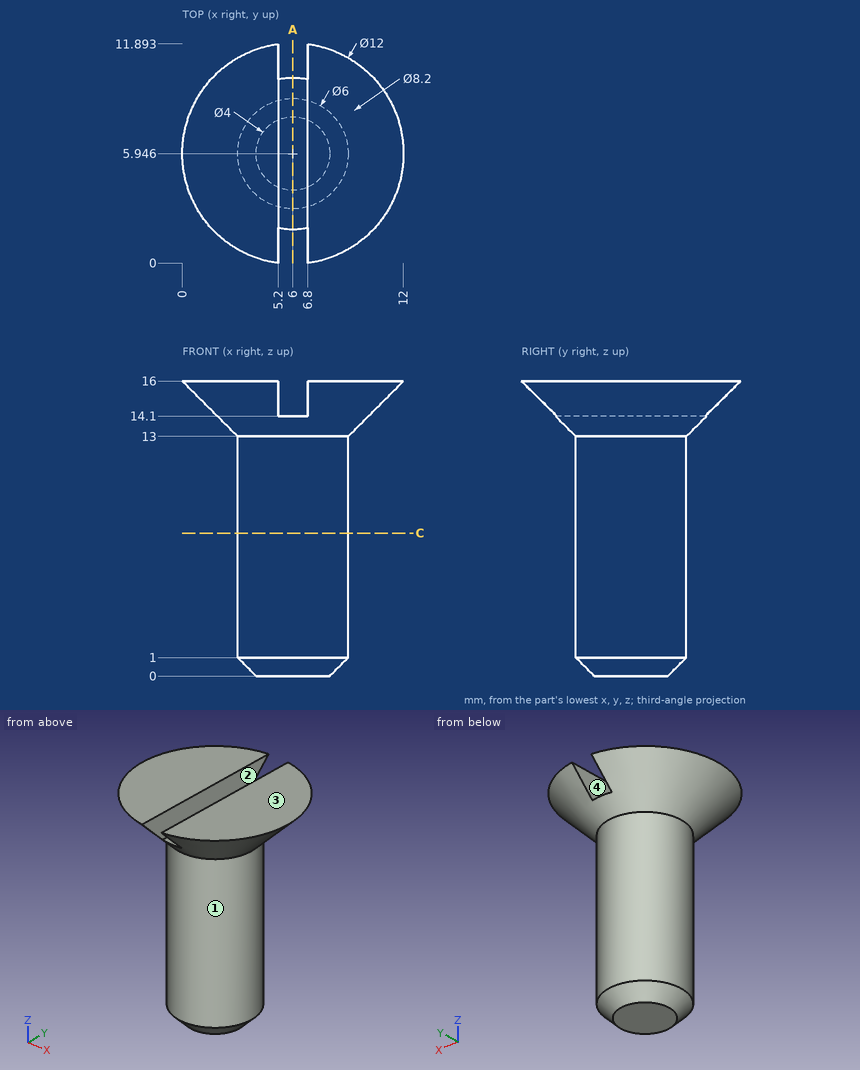
Drawing for the job (mm, zero at the part's lowest x, y, z). Round coordinates to 2 decimals unless told otherwise and drop trailing zeros. Write each loop counter-clockwise with the first axis right and the second up, starting at its lowest first coordinate (ties: lowest second). Pieces come first, ordered by that corner, then holes. Notation, with made-up numbers: M 34,84.25 L 55,84.25 A18 cw 55,92.25 Z; hole C 14,44.25 d3. An arc over 180 degrees is marked long. Answer as a JSON object with one key per item and string values. Group by question number.
(1) Mould opens along X. For the marked faces 1, 2, 3 and 4 say: pulls with the +X half, pulls with the -X half, needs draft (parallel to the pull), parting line crosses it, or undercut.
(2) Cut at C-C (z = 7.75). Give the cut face in (x, y).
(3) Drill centre lines: L1, parallel to Y at x = 4.75, z = 13.25 (1 decimal); L2, parallel to Z at x = 2.5, y = 9 (1 decimal); L3, parallel to Z at x = 7.25, y = 3.75 (1 decimal). Where is each one in solid material? Low to high.
(4) Cut at A-A (x = 6). Give the cut face in (y, z), and give its area (3 significant figures).
(5) Flat gauge pins, fed straight in: pin 1 (1.3 mm diameter, centred on x = 6, y = 4, fed in from +Z); pin 2 (1 mm diameter, centred on y = 4, z = 15.5, fed in from +X); pin 3 (0.6 mm diameter, centred on y = 9, z = 15, fed in from -X) (1 decimal). Where does each tip first touch, or does it go through?
Responses:
{
 "1": {"face 1": "parting line crosses it", "face 2": "undercut", "face 3": "needs draft", "face 4": "undercut"},
 "2": {"outline": "C 6,5.95 d6"},
 "3": {"L1": "y = 2.9 to 8.9", "L2": "z = 14.6 to 16", "L3": "z = 0.5 to 16"},
 "4": {"outline": "M 1.85,14.1 L 2.95,13 L 2.95,1 L 3.95,0 L 7.95,0 L 8.95,1 L 8.95,13 L 10.05,14.1 Z", "area": "84.8 mm2"},
 "5": {"pin 1": "stops at z = 14.1", "pin 2": "stops at x = 11.7", "pin 3": "stops at x = 1.6"}
}
